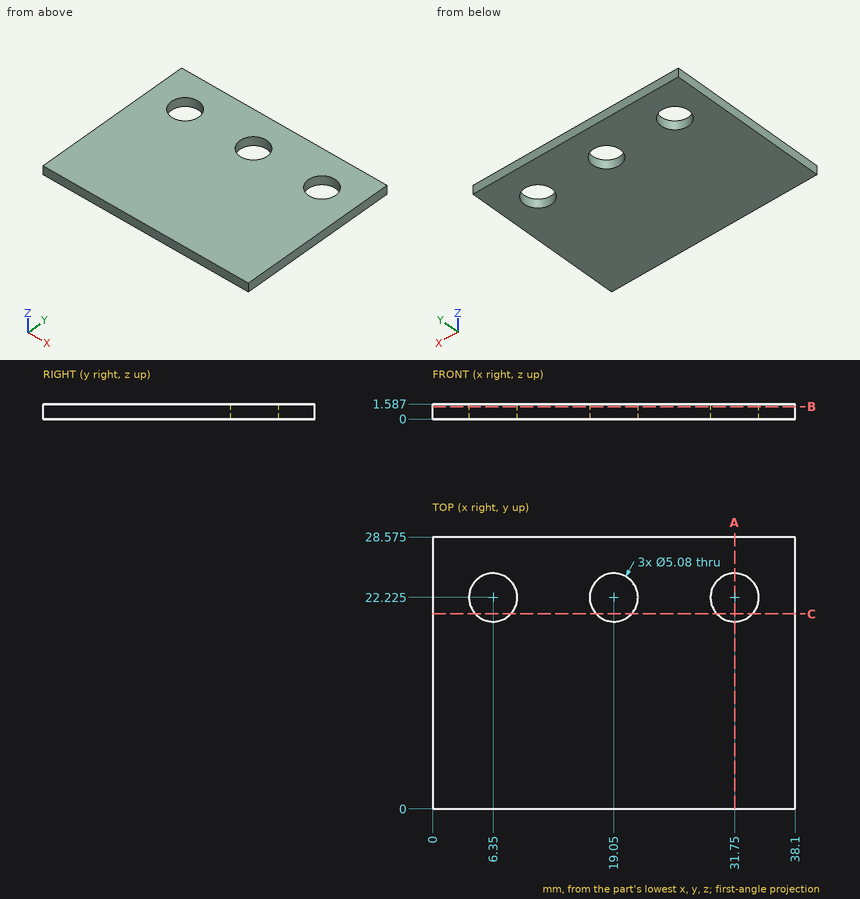
Study the drawing (mm; zero at the part's minimum x, y, z) and answer. Round coordinates to 2 decimals unless told otherwise and drop trailing zeros. Write each loop counter-clockwise with the first axis right and the second up, starting at its lowest first coordinate (ties: lowest second). Pieces come first, ordered by that corner, then holes.
Q1. A flat-ended cylindrical pin translates along its axis: P1, Ø6, axis at x = 6.35, y = 22.225, coming from the -Z side. Find the tip coordinate at first contact, or state that the pin passes through.
Values:
P1: stops at z = 0
Q2. Find section C-C on y = 20.5. Determine the outline of the cut face in (x, z) (1 decimal).
Values:
outline: (0, 0) - (4.5, 0) - (4.5, 1.6) - (0, 1.6) - close; (8.2, 0) - (17.2, 0) - (17.2, 1.6) - (8.2, 1.6) - close; (20.9, 0) - (29.9, 0) - (29.9, 1.6) - (20.9, 1.6) - close; (33.6, 0) - (38.1, 0) - (38.1, 1.6) - (33.6, 1.6) - close
Q3. Find section B-B on z = 1.3. State how many separate pieces and enclosed holes the cut face has, and give its area (3 significant figures).
Values:
separate pieces: 1
enclosed holes: 3
area: 1,030 mm2
Q4. Straight lines are drawn through the part: line 1 (Y direction, x = 6.35, z = 0.75) (1 decimal); line 2 (X direction, y = 20, z = 1.4) (1 decimal); line 3 (Y direction, x = 32.5, z = 0.9) (1 decimal). For each, find the intervals that lie inside material, in ascending order.
Values:
line 1: y = 0 to 19.7, 24.8 to 28.6
line 2: x = 0 to 5.1, 7.6 to 17.8, 20.3 to 30.5, 33 to 38.1
line 3: y = 0 to 19.8, 24.7 to 28.6
Q5. Find section A-A on x = 31.75. Determine the outline of the cut face in (y, z) (1 decimal).
Values:
outline: (0, 0) - (19.7, 0) - (19.7, 1.6) - (0, 1.6) - close; (24.8, 0) - (28.6, 0) - (28.6, 1.6) - (24.8, 1.6) - close
